```python
from build123d import *

# Parameters (mm, degrees)
SKETCH_1_R               = 30
SKETCH_1_R_2             = 2.5
SKETCH_1_R_3             = 5.25
EXTRUDE_1_DEPTH          = 6
SKETCH_3_R               = 11.25
SKETCH_3_R_2             = 5.25
EXTRUDE_2_DEPTH          = 20.4
SKETCH_4_R               = 1.5
CUT_EXTRUDE_1_DEPTH      = 31
CUT_EXTRUDE_1_DEPTH_BACK = 31


with BuildPart() as part:
    # ｽｹｯﾁ1 → ﾎﾞｽ - 押し出し1 (new body)
    with BuildSketch(Plane.XY):
        Circle(SKETCH_1_R)
        with Locations((-23.5, 0)):
            Circle(SKETCH_1_R_2, mode=Mode.SUBTRACT)
        with Locations((11.75, -20.351596989)):
            Circle(SKETCH_1_R_2, mode=Mode.SUBTRACT)
        with Locations((11.75, 20.351596989)):
            Circle(SKETCH_1_R_2, mode=Mode.SUBTRACT)
        Circle(SKETCH_1_R_3, mode=Mode.SUBTRACT)
    extrude(amount=EXTRUDE_1_DEPTH)

    # ｽｹｯﾁ3 → ﾎﾞｽ - 押し出し2 (add)
    with BuildSketch(Plane.XY.offset(6)):
        Circle(SKETCH_3_R)
        Circle(SKETCH_3_R_2, mode=Mode.SUBTRACT)
    extrude(amount=EXTRUDE_2_DEPTH)

    # ｽｹｯﾁ4 → ｶｯﾄ - 押し出し1 (cut, two sides)
    with BuildSketch(Plane(origin=(0, 0, 0), x_dir=(1, 0, 0), z_dir=(0, 1, 0))) as cut_extrude_1_sk:
        with Locations((0, -16.2)):
            Circle(SKETCH_4_R)
    extrude(amount=CUT_EXTRUDE_1_DEPTH, mode=Mode.SUBTRACT)
    extrude(cut_extrude_1_sk.sketch, amount=-CUT_EXTRUDE_1_DEPTH_BACK, mode=Mode.SUBTRACT)


solid = part.part
```
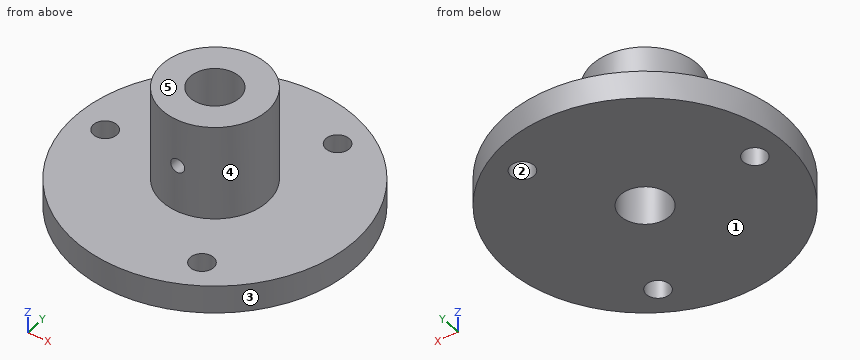
For this review, take the finished solid that the model builds, in its own axes (mm). Face numbers are marked on the shaded views. A direction names the side the tool comes from. Coordinates: 2 decimals unless noted, no trailing zeros. Write each loop counter-clockwise with the first axis right and the second up, starting at its lowest first coordinate (ties: lowest second). Pieces come first, ordered by that corner, then holes.
(1) Wall thickness on probe 1 along Y at (x, z) = (11.75, 4.45); probe 2 along Z at (x, y) = (20, -22); probe 3 along Z at (x, y) = (0, -8): over which ranges is each line inside the solid? List them lowest first.
(2) Add section A-A on x = 0. Give the boundary of the cut face in (y, z), then the cut area to 3 significant figures.
(3) For pin 1 Ø12 at (x, z) = (22, 17) entering from +Y; pin 2 Ø5 at (y, z) = (3.5, 21.5) entering from -X; pin 3 Ø5 at (x, z) = (-12.5, 8) entering from +Y, all flat-tipped, find the tip position at first contact; note any pin that passes through.
(4) Add section B-B on y = 0. Give the boundary of the cut face in (x, z).
(5) Add section D-D on x = -23.5. Give the boundary of the cut face in (y, z).
(6) Tool access review of the marked faces 4 and 5: name each direction out of +Z, -Z, +X, -X, +Y, -Y from which nothing blocks a thin tool from reaching the whole face with its end or side.
(7) The part is to be moulded in two halves that separate along Y. For the marked faces 1, 2 and 3, say which applies: +Y half, -Y half, draft (parallel to the pull), parting line (faces both ways), or undercut.
(8) Add section C-C on z = 16.2. Give the boundary of the cut face in (x, y), then the cut area to 3 significant figures.
Answer sheet:
1. probe 1: y = -27.6 to -22.85, -17.85 to 17.85, 22.85 to 27.6
1. probe 2: z = 0 to 6
1. probe 3: z = 0 to 14.7, 17.7 to 26.4
2. outline: (-30, 0) - (-5.25, 0) - (-5.25, 14.7) - (-11.25, 14.7) - (-11.25, 6) - (-30, 6) - close; (-11.25, 17.7) - (-5.25, 17.7) - (-5.25, 26.4) - (-11.25, 26.4) - close; (5.25, 0) - (30, 0) - (30, 6) - (11.25, 6) - (11.25, 14.7) - (5.25, 14.7) - close; (5.25, 17.7) - (11.25, 17.7) - (11.25, 26.4) - (5.25, 26.4) - close
2. area: 506 mm2
3. pin 1: passes through
3. pin 2: stops at x = -11.21
3. pin 3: stops at y = 27.91
4. outline: (-30, 0) - (-26, 0) - (-26, 6) - (-30, 6) - close; (-21, 0) - (-5.25, 0) - (-5.25, 26.4) - (-11.25, 26.4) - (-11.25, 6) - (-21, 6) - close; (5.25, 0) - (30, 0) - (30, 6) - (11.25, 6) - (11.25, 26.4) - (5.25, 26.4) - close
5. outline: (-18.65, 0) - (-2.5, 0) - (-2.5, 6) - (-18.65, 6) - close; (2.5, 0) - (18.65, 0) - (18.65, 6) - (2.5, 6) - close
6. face 4: +Z
6. face 5: +Z, +X, -X, +Y, -Y
7. face 1: draft
7. face 2: undercut
7. face 3: parting line
8. outline: (-1.5, -11.15) - (-1.5, -5.03) arc R5.25 cw to (-1.5, 5.03) - (-1.5, 11.15) arc R11.25 ccw to start; (1.5, -11.15) arc R11.25 ccw to (1.5, 11.15) - (1.5, 5.03) arc R5.25 cw to (1.5, -5.03) - close
8. area: 275 mm2
